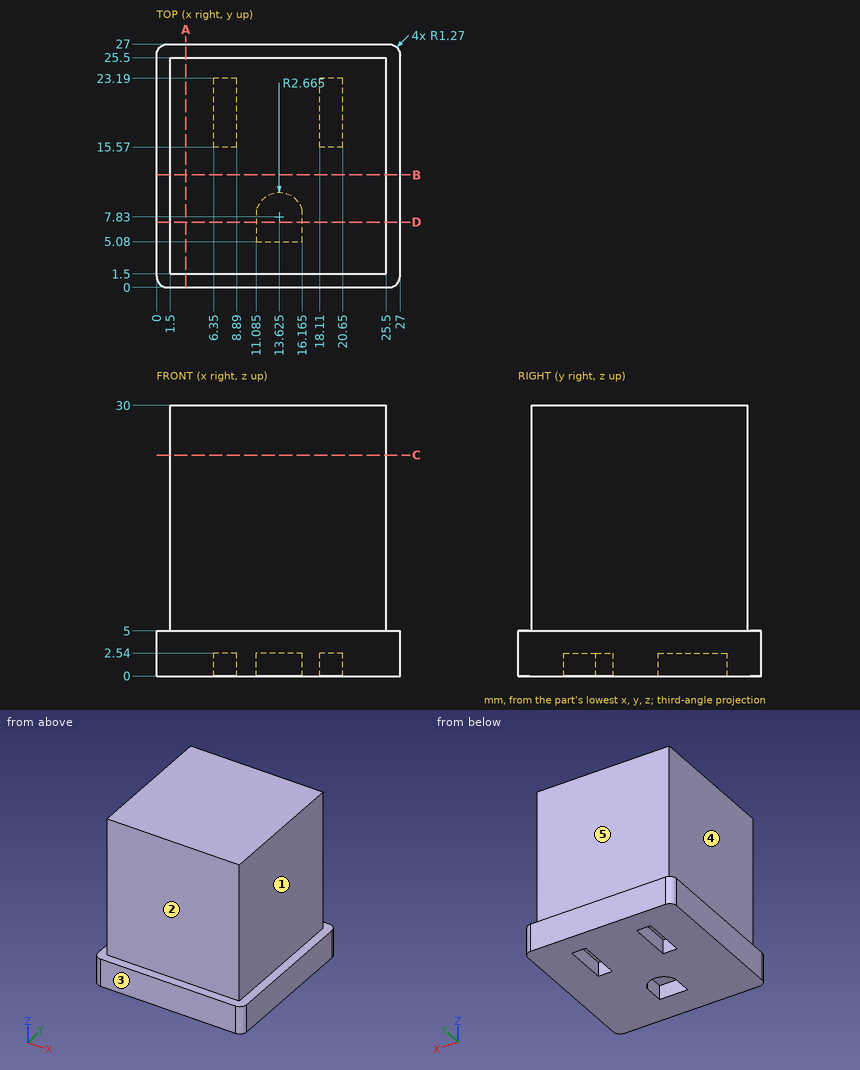
For this review, use the dimensioned drawing (mm, ordinates from the lowest corner) and the shaded views. A direction names the side the tool comes from. Coordinates: 2 decimals unless noted, no trailing zeros. Loops run counter-clockwise (first coordinate to the right, second up) from the corner with the lowest first, then second, coordinate; pieces in that order, holes last. Notation, with made-up numbers: (13.5, 56) -> (24.5, 56) arc R32 ccw to (24.5, 87) -> close; hole circle Ø2 at (74, 86). An arc over 180 degrees is marked (long way). Use a Markdown table: item, result. Add a question column.
Item 1: We need section C-C, the plane z = 24.5. Write out the cut boundary in (x, y), and give its area (3 significant figures).
Item 2: We need section D-D, the plane y = 7.25. Write out the cut boundary in (x, z) (1 decimal), and give its area (3 significant figures).
Item 3: Machinability: for the marked faces 1, 2, 3, 4 and 5, which of the approach directions +Z, -Z, +X, -X, +Y, -Y give a long, thin tool a straight path to every point of the face, cutting with its end or side? Answer none if there is none.
Item 4: We need section A-A, the plane x = 3.25. Write out the cut boundary in (y, z).
Item 5: Clearance check with flat-ended pins moving along their axes: P1, Ø1.3, axis at x = 19, y = 21, coming from the -Z side; P2, Ø4, axis at y = 18, z = 24.5, coming from the +X side; P3, Ø3, axis at y = 22.5, z = 16, coming from the -X side. State where each tip first meets the part, or that it passes through.
Item 6: Wall thickness on L1, parallel to X at y = 20.5, z = 1.5; L2, parallel to X at y = 20, z = 22.5: over which ranges is each line inside the solid? List them lowest first. Write a range as from..to.
Numbers:
| question | item | result |
|---|---|---|
| 1 | outline | (1.5, 1.5) -> (25.5, 1.5) -> (25.5, 25.5) -> (1.5, 25.5) -> close |
| 1 | area | 576 mm^2 |
| 2 | outline | (0, 0) -> (11.1, 0) -> (11.1, 2.5) -> (16.2, 2.5) -> (16.2, 0) -> (27, 0) -> (27, 5) -> (25.5, 5) -> (25.5, 30) -> (1.5, 30) -> (1.5, 5) -> (0, 5) -> close |
| 2 | area | 722 mm^2 |
| 3 | face 1 | +Z, +X, +Y, -Y |
| 3 | face 2 | +Z, +X, -X, -Y |
| 3 | face 3 | +Z, -Z, +X, -X, -Y |
| 3 | face 4 | +Z, -X, +Y, -Y |
| 3 | face 5 | +Z, +X, -X, +Y |
| 4 | outline | (0, 0) -> (27, 0) -> (27, 5) -> (25.5, 5) -> (25.5, 30) -> (1.5, 30) -> (1.5, 5) -> (0, 5) -> close |
| 5 | P1 | stops at z = 2.54 |
| 5 | P2 | stops at x = 25.5 |
| 5 | P3 | stops at x = 1.5 |
| 6 | L1 | x = 0..6.35, 8.89..18.11, 20.65..27 |
| 6 | L2 | x = 1.5..25.5 |
